Source: CAD feature listing. Evaluate the final solid. Frame: model axes, mm. Face numbers are marked on the shaded views. A direction names the side the tool comes from. Round coordinates to 2 decimals unless told otherwise and drop trailing zeros. Order: outer loops, then holes, each group sorted by start corner. A loop starts at its lowest first (then second) coordinate and runs counter-clockwise, first axis right, second up. Notation, with made-up numbers: (-38, -18.75) -> (2, -18.75) arc R13 ccw to (2, 0.25) -> close; hole circle Ø9 at (36.5, -12). An arc over 180 degrees is marked (long way). One line per item, written item: value. Start each with the question number.
1) Mould query, pull axis Y, two halves, no side actions, for the marked faces 3, 4 and 5. Classes: pulls with the +Y half, pulls with the -Y half, needs draft (parallel to the pull), parting line crosses it, or undercut.
2) Pin query (flat end, axial travel): P1, Ø10, axis at y = 29, z = -0.5, coming from the -X side; P2, Ø4, axis at x = 9.5, y = 21, coming from the -Z side; P3, Ø12, axis at x = 7.5, z = -0.5, coming from the +Y side; P4, Ø4, axis at x = -5, y = 44.5, coming from the +Z side. Return the tip coordinate at first contact, or that it passes through.
3) Reachability of the marked faces 1 and 2 from +Z, -Z, +X, -X, +Y, -Y: full face, straight path, thin tool, end or side. Return the list, or none.
4) Section D-D (x = -15.5). Return the cut outline in (y, z), and give its area (3 significant figures).
5) Ray query, L1, parallel to Z at x = 15.5, y = 44.7; L2, parallel to X at y = 46, z = -15. Return the intervals inside material, ascending.
```python
from build123d import *

# Parameters (mm, degrees)
SKETCH1_W               = 42.3
SKETCH1_H               = 42.3
BOSS_EXTRUDE1_DEPTH     = 48
SKETCH2_R               = 11
BOSS_EXTRUDE2_DEPTH     = 2
SKETCH3_R               = 2.5
BOSS_EXTRUDE3_DEPTH     = 16
CUT_EXTRUDE1_DEPTH      = 19
CUT_EXTRUDE1_DEPTH_BACK = 49
SKETCH5_W               = 33.814718626
SKETCH5_H               = 24
CUT_EXTRUDE2_DEPTH      = 0.01
CUT_EXTRUDE3_START      = -12
CUT_EXTRUDE3_DEPTH      = 24
CIRPATTERN1_COUNT       = 4
SKETCH7_R               = 1.5
CUT_EXTRUDE4_DEPTH      = 4.5
SKETCH8_W               = 16
SKETCH8_H               = 11
BOSS_EXTRUDE4_DEPTH     = 6
SKETCH9_W               = 16
SKETCH9_H               = 5
CUT_EXTRUDE5_DEPTH      = 2.5
FILLET1_R               = 1.5
SKETCH10_W              = 13
SKETCH10_H              = 4.5
CUT_EXTRUDE6_DEPTH      = 5
CUT_EXTRUDE7_DEPTH      = 30.15
BOSS_EXTRUDE5_DEPTH     = 4
SKETCH13_W              = 16
SKETCH13_H              = 0.25
CUT_EXTRUDE8_DEPTH      = 0.5
FILLET2_R               = 0.125


with BuildPart() as part:
    # Sketch1 → Boss-Extrude1 (new body)
    with BuildSketch(Plane(origin=(0, 0, 0), x_dir=(1, 0, 0), z_dir=(0, 1, 0))):
        Rectangle(SKETCH1_W, SKETCH1_H)
    extrude(amount=BOSS_EXTRUDE1_DEPTH)

    # Sketch2 → Boss-Extrude2 (add)
    with BuildSketch(Plane(origin=(0, 48, 0), x_dir=(1, 0, 0), z_dir=(0, 1, 0))):
        Circle(SKETCH2_R)
    extrude(amount=BOSS_EXTRUDE2_DEPTH)

    # Sketch3 → Boss-Extrude3 (add)
    with BuildSketch(Plane(origin=(0, 50, 0), x_dir=(1, 0, 0), z_dir=(0, 1, 0))):
        Circle(SKETCH3_R)
    extrude(amount=BOSS_EXTRUDE3_DEPTH)

    # Sketch4 → Cut-Extrude1 (cut, two sides)
    with BuildSketch(Plane(origin=(0, 48, 0), x_dir=(1, 0, 0), z_dir=(0, 1, 0))) as cut_extrude1_sk:
        Polygon((-21.15, 16.907359313), (-16.907359313, 21.15), (-21.15, 21.15), align=None)
        Polygon((21.15, 21.15), (21.15, 16.907359313), (16.907359313, 21.15), align=None)
        Polygon((21.15, -16.907359313), (16.907359313, -21.15), (21.15, -21.15), align=None)
        Polygon((-21.15, -21.15), (-21.15, -16.907359313), (-16.907359313, -21.15), align=None)
    extrude(amount=CUT_EXTRUDE1_DEPTH, mode=Mode.SUBTRACT)
    extrude(cut_extrude1_sk.sketch, amount=-CUT_EXTRUDE1_DEPTH_BACK, mode=Mode.SUBTRACT)

    # Sketch5 → Cut-Extrude2 (cut)
    with BuildSketch(Plane(origin=(21.15, 0, 0), x_dir=(0, 0, -1), z_dir=(1, 0, 0))):
        with Locations((0, 24)):
            Rectangle(SKETCH5_W, SKETCH5_H)
    cut_extrude2 = extrude(amount=-CUT_EXTRUDE2_DEPTH, mode=Mode.SUBTRACT)

    # Sketch6 → Cut-Extrude3 (cut)
    with BuildSketch(Plane(origin=(0, 48, 0), x_dir=(1, 0, 0), z_dir=(0, 1, 0)).offset(CUT_EXTRUDE3_START)):
        Polygon((21.15, 14.078932188), (14.078932188, 21.15), (21.15, 21.15), align=None)
    cut_extrude3 = extrude(amount=-CUT_EXTRUDE3_DEPTH, mode=Mode.SUBTRACT)

    # CirPattern1: Cut-Extrude2, Cut-Extrude3 ×4 about axis
    cirpattern1_axis = Axis((0, 0, 0), (0, 1, 0))
    for i in range(1, CIRPATTERN1_COUNT):
        add(cut_extrude2.rotate(cirpattern1_axis, i * 360 / CIRPATTERN1_COUNT), mode=Mode.SUBTRACT)
        add(cut_extrude3.rotate(cirpattern1_axis, i * 360 / CIRPATTERN1_COUNT), mode=Mode.SUBTRACT)

    # Sketch7 → Cut-Extrude4 (cut)
    with BuildSketch(Plane(origin=(0, 48, 0), x_dir=(1, 0, 0), z_dir=(0, 1, 0))):
        with Locations((15.5, 15.5)):
            Circle(SKETCH7_R)
        with Locations((15.5, -15.5)):
            Circle(SKETCH7_R)
        with Locations((-15.5, -15.5)):
            Circle(SKETCH7_R)
        with Locations((-15.5, 15.5)):
            Circle(SKETCH7_R)
    extrude(amount=-CUT_EXTRUDE4_DEPTH, mode=Mode.SUBTRACT)

    # Sketch8 → Boss-Extrude4 (add)
    with BuildSketch(Plane.XY.offset(21.15)):
        with Locations((0, 5.5)):
            Rectangle(SKETCH8_W, SKETCH8_H)
    extrude(amount=BOSS_EXTRUDE4_DEPTH)

    # Sketch9 → Cut-Extrude5 (cut)
    with BuildSketch(Plane.XY.offset(27.15)):
        with Locations((0, 2.5)):
            Rectangle(SKETCH9_W, SKETCH9_H)
    extrude(amount=-CUT_EXTRUDE5_DEPTH, mode=Mode.SUBTRACT)

    # Fillet1
    fillet1_edges = [part.edges().sort_by_distance(p)[0] for p in [
        (0, 0, 24.65),
    ]]
    fillet(fillet1_edges, radius=FILLET1_R)

    # Sketch10 → Cut-Extrude6 (cut)
    with BuildSketch(Plane(origin=(0, 11, 0), x_dir=(1, 0, 0), z_dir=(0, 1, 0))):
        with Locations((0, -24.9)):
            Rectangle(SKETCH10_W, SKETCH10_H)
    extrude(amount=-CUT_EXTRUDE6_DEPTH, mode=Mode.SUBTRACT)

    # Sketch11 → Cut-Extrude7 (cut, through all)
    with BuildSketch(Plane(origin=(8, 0, 0), x_dir=(0, 0, -1), z_dir=(1, 0, 0))):
        with BuildLine():
            Line((-27.15, 9.5), (-25.15, 9.5))
            ThreePointArc((-25.15, 9.5), (-24.65, 9), (-25.15, 8.5))
            Line((-25.15, 8.5), (-27.15, 8.5))
            Line((-27.15, 8.5), (-27.15, 9.5))
        make_face()
    extrude(amount=-CUT_EXTRUDE7_DEPTH, mode=Mode.SUBTRACT)

    # Sketch12 → Boss-Extrude5 (add)
    with BuildSketch(Plane(origin=(0, 6, 0), x_dir=(1, 0, 0), z_dir=(0, 1, 0))):
        with BuildLine():
            Line((-2.667, -22.65), (-2.167, -22.65))
            Line((-2.167, -22.65), (-2.167, -26.4))
            ThreePointArc((-2.167, -26.4), (-2.417, -26.65), (-2.667, -26.4))
            Line((-2.667, -26.4), (-2.667, -22.65))
        make_face()
        with BuildLine():
            Line((5.334, -22.65), (5.334, -26.4))
            ThreePointArc((5.334, -26.4), (5.084, -26.65), (4.834, -26.4))
            Line((4.834, -26.4), (4.834, -22.65))
            Line((4.834, -22.65), (5.334, -22.65))
        make_face()
        with BuildLine():
            Line((-4.834, -22.65), (-5.334, -22.65))
            Line((-5.334, -22.65), (-5.334, -26.4))
            ThreePointArc((-5.334, -26.4), (-5.084, -26.65), (-4.834, -26.4))
            Line((-4.834, -26.4), (-4.834, -22.65))
        make_face()
        with BuildLine():
            Line((2.167, -22.65), (2.167, -26.4))
            ThreePointArc((2.167, -26.4), (2.417, -26.65), (2.667, -26.4))
            Line((2.667, -26.4), (2.667, -22.65))
            Line((2.667, -22.65), (2.167, -22.65))
        make_face()
    extrude(amount=BOSS_EXTRUDE5_DEPTH)

    # Sketch13 → Cut-Extrude8 (cut)
    with BuildSketch(Plane(origin=(0, 11, 0), x_dir=(1, 0, 0), z_dir=(0, 1, 0))):
        with Locations((0, -21.275)):
            Rectangle(SKETCH13_W, SKETCH13_H)
    extrude(amount=-CUT_EXTRUDE8_DEPTH, mode=Mode.SUBTRACT)

    # Fillet2
    fillet2_edges = [part.edges().sort_by_distance(p)[0] for p in [
        (0, 10.5, 21.4),
    ]]
    fillet(fillet2_edges, radius=FILLET2_R)


solid = part.part
```
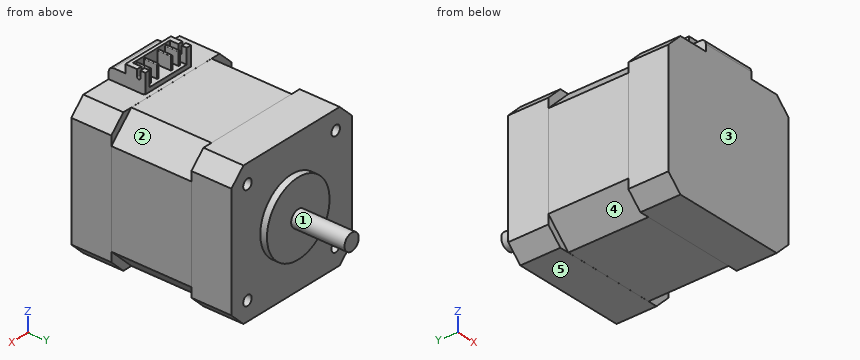
Findings:
1. face 3: pulls with the -Y half
1. face 4: undercut
1. face 5: needs draft
2. P1: x = -21.14
2. P2: z = -21.14
2. P3: y = 66
2. P4: z = 21.15
3. face 1: +Y
3. face 2: +Z, +X
4. outline: (0, -21.15) -> (12, -21.15) -> (12, -19.73) -> (36, -19.73) -> (36, -21.15) -> (48, -21.15) -> (48, -17) -> (43.5, -17) -> (43.5, -14) -> (48, -14) -> (48, 14) -> (43.5, 14) -> (43.5, 17) -> (48, 17) -> (48, 21.15) -> (36, 21.15) -> (36, 19.73) -> (12, 19.73) -> (12, 21.15) -> (0, 21.15) -> close
4. area: 1,940 mm2
5. L1: -21.15 to -17, -14 to 14, 17 to 21.15
5. L2: -21.15 to -16.91, -14.09 to 14.09, 16.91 to 21.15
